```python
from build123d import *

# Parameters (mm, degrees)
CYLINDER003_R     = 2
CYLINDER003_DEPTH = 16
CYLINDER004_R     = 4
CYLINDER004_DEPTH = 14
BOX001_W          = 30
BOX001_H          = 10
BOX001_DEPTH      = 10
FILLET002_R       = 1
BOX002_W          = 10
BOX002_H          = 30
BOX002_DEPTH      = 20


with BuildPart() as part:
    # Cone → Cone (revolve)
    with BuildSketch(Plane.XZ):
        Polygon((0, 0), (10, 0), (5, 16), (0, 16), align=None)
    revolve(axis=Axis((0, 0, 0), (0, 0, 1)))

    # Cylinder003 → Cylinder003 (cut)
    with BuildSketch(Plane.XY):
        Circle(CYLINDER003_R)
    extrude(amount=CYLINDER003_DEPTH, mode=Mode.SUBTRACT)

    # Cylinder004 → Cylinder004 (cut)
    with BuildSketch(Plane.XY):
        Circle(CYLINDER004_R)
    extrude(amount=CYLINDER004_DEPTH, mode=Mode.SUBTRACT)

    # Box001 → Box001 (cut)
    with BuildSketch(Plane(origin=(-15, 3.5, -7), x_dir=(1, 0, 0), z_dir=(0, 0.190809, 0.981627))):
        with Locations((15, 5)):
            Rectangle(BOX001_W, BOX001_H)
    extrude(amount=BOX001_DEPTH, mode=Mode.SUBTRACT)

    # Fillet002
    fillet002_edges = [part.edges().sort_by_distance(p)[0] for p in [
        (-5, 0, 16),
    ]]
    fillet(fillet002_edges, radius=FILLET002_R)

    # Box002 → Box002 (cut)
    with BuildSketch(Plane(origin=(7, -15, 0), x_dir=(1, 0, 0), z_dir=(0, 0, 1))):
        with Locations((5, 15)):
            Rectangle(BOX002_W, BOX002_H)
    extrude(amount=BOX002_DEPTH, mode=Mode.SUBTRACT)


with BuildPart() as part_1:
    # Body001 placement: moved
    add(part.part.moved(Location((-18, 0, 0))))


solid = part_1.part
```
Check sheet for the modelled part. Datum: model origin and axes. Units: mm. A direction names the side the tool comes from. Give positions to 0.01 mm unless a question says otherwise; leave off trailing zeros. Order: outer loops, then holes, each group sorted by start corner. A loop starts at its lowest first (then second) coordinate and runs counter-clockwise, first axis right, second up. Notation, with made-up numbers: (79.25, 68) -> (100.25, 68) arc R30 ccw to (100.25, 90) -> close; hole circle Ø1 at (29.5, 40). An arc over 180 degrees is marked (long way). Return JSON: item names as keys, results as strings.
1. Mould release check, pull along X, two halves, no side actions. Record for faces 1 (the flat face through (-18.98, 5.13, 1.39)), 2 (the cylindrical face through (-21.2, -2.4, 6.9)), 3 (the conical face through (-23.17, -3.96, 11.16)): +X half, -X half, draft (parallel to the pull), parting line (faces both ways), or undercut.
From the geometry:
{"face 1": "draft", "face 2": "undercut", "face 3": "parting line"}
2. Cross-section at D-D, the plane z = 7. Record the cut outline in (x, y) (1 decimal), plus the area to 3 significant figures.
From the geometry:
{"outline": "(-11, -3.5) -> (-11, 3.5) arc R7.8 ccw (long way) to start; hole circle Ø8 at (-18, 0)", "area": "138 mm^2"}
3. Cross-section at C-C, the plane z = 12. Record the cut outline in (x, y).
From the geometry:
{"outline": "circle Ø12.5 at (-18, 0); hole circle Ø8 at (-18, 0)"}
4. Cross-section at A-A, the plane x = -18. Record the cut outline in (y, z).
From the geometry:
{"outline": "(-10, 0) -> (-4, 0) -> (-4, 14) -> (-2, 14) -> (-2, 16) -> (-4.26, 16) arc R1 ccw to (-5.22, 15.3) -> close; (2, 14) -> (4, 14) -> (4, 0) -> (4.86, 0) -> (5.41, 2.82) -> (9.36, 2.05) -> (5.22, 15.3) arc R1 ccw to (4.26, 16) -> (2, 16) -> close"}
5. Material ranges on probe 1 along Y at (x, z) = (-18, 14.85); probe 2 along Y at (x, z) = (-18, 5.25); probe 3 along Z at (x, y) = (-14.75, -0.25), recorded low to high. Write a range as [from, to].
From the geometry:
{"probe 1": "[-5.36, -2], [2, 5.36]", "probe 2": "[-8.36, -4], [4, 8.36]", "probe 3": "[14, 16]"}
6. Cross-section at B-B, the plane y = 0. Record the cut outline in (x, z).
From the geometry:
{"outline": "(-28, 0) -> (-22, 0) -> (-22, 14) -> (-20, 14) -> (-20, 16) -> (-22.26, 16) arc R1 ccw to (-23.22, 15.3) -> close; (-16, 14) -> (-14, 14) -> (-14, 0) -> (-11, 0) -> (-11, 9.6) -> (-12.78, 15.3) arc R1 ccw to (-13.74, 16) -> (-16, 16) -> close"}
7. Set-up check for faces 4 (the flat face through (-18.272, 6.973, 2.512)), 5 (the flat face through (-20, -1, 14)), 6 (the flat face through (-19.4, -4.1, 0)): record each of +Z, -Z, +X, -X, +Y, -Y from which the full face is reachable in a straight line by a thin tool's end or side.
From the geometry:
{"face 4": "-Z, +X, -X", "face 5": "-Z", "face 6": "-Z, +X, -X, +Y, -Y"}
8. Go/stop test with flat-tipped pins: P1, Ø3.5, axis at x = -18, y = 0, coming from the -Z side; P2, Ø3, axis at x = -13, z = 8.5, coming from the -Y side; P3, Ø4, axis at x = -16.5, y = -0.5, coming from the -Z side; P4, Ø5, axis at x = -18, y = 0, coming from the +Z side. Record where each tip stops, or that it passes through.
From the geometry:
{"P1": "through", "P2": "y = -6.61", "P3": "z = 14", "P4": "z = 16"}
